Geometry: see drawing. Coordinates: mm, zero at the bounding-box minimum. Coordinates: 2 decimals unless noted, no trailing zeros. Write each loop counter-clockwise with the first axis right and the second up, starting at its lowest first coordinate (ties: lowest second). Pieces come first, ordered by that corner, then holes. Notation, with made-up numbers: (24.5, -2.75) - (47.5, -2.75) arc R27 cw to (47.5, 22.25) - close; hole circle Ø1 at (13.25, -27.5). An arc over 180 degrees is marked (long way). One line per question, with ' | ' between items. Start each with the question number.
Q1. Cut plane A-A, the plane y = 100. Return loops of the section in (x, z).
Q2. Line query: line 1 (Y direction, x = 68.5, z = 1.75) (1 decimal); line 2 (Y direction, x = 67, z = 1); line 3 (Y direction, x = 36, z = 9.5). Output: solid intervals per line, ascending.
Q3. Cut plane B-B, the plane z = 7.5. Return loops of the section in (x, y), plus the area to 3 significant figures.
Q4. Cut plane C-C, the plane x = 67. Return loops of the section in (y, z).
Q5. Cut plane D-D, the plane y = 53. Return loops of the section in (x, z) (1 decimal).
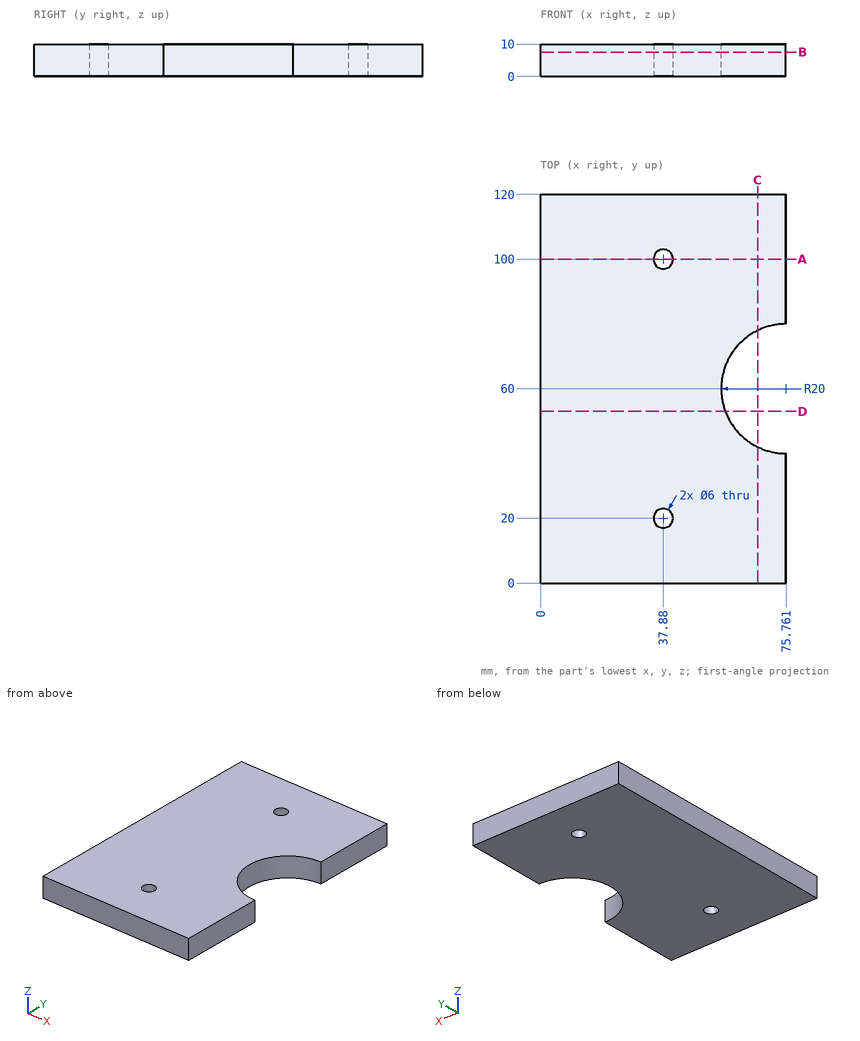
Reply:
1) outline: (0, 0) - (34.88, 0) - (34.88, 10) - (0, 10) - close; (40.88, 0) - (75.76, 0) - (75.76, 10) - (40.88, 10) - close
2) line 1: y = 0 to 41.4, 78.6 to 120 | line 2: y = 0 to 42.02, 77.98 to 120 | line 3: y = 0 to 17.66, 22.34 to 97.66, 102.34 to 120
3) outline: (0, 0) - (75.76, 0) - (75.76, 40) arc R20 cw to (75.76, 80) - (75.76, 120) - (0, 120) - close; hole circle Ø6 at (37.88, 20); hole circle Ø6 at (37.88, 100) | area: 8,410 mm^2
4) outline: (0, 0) - (42.02, 0) - (42.02, 10) - (0, 10) - close; (77.98, 0) - (120, 0) - (120, 10) - (77.98, 10) - close
5) outline: (0, 0) - (57, 0) - (57, 10) - (0, 10) - close
